Print and shaded views of the part. All mm, measured from the part's lowest x, y and z. A direction names the side the tool comes from. Give positions to 0.01 mm unless a question says otherwise; leave off trailing zeros. Write each loop counter-clockwise with the first axis right and the second up, starting at its lowest first coordinate (ties: lowest second). Pieces come first, ordered by that corner, then holes. Notation, with made-up numbers: (-39.75, -28) - (-13.75, -28) arc R21 ccw to (-13.75, -3) - close; hole circle Ø5 at (1, 78). An arc over 180 degrees is marked (long way). Use one line per item in the form item = value. Start each with the question number.
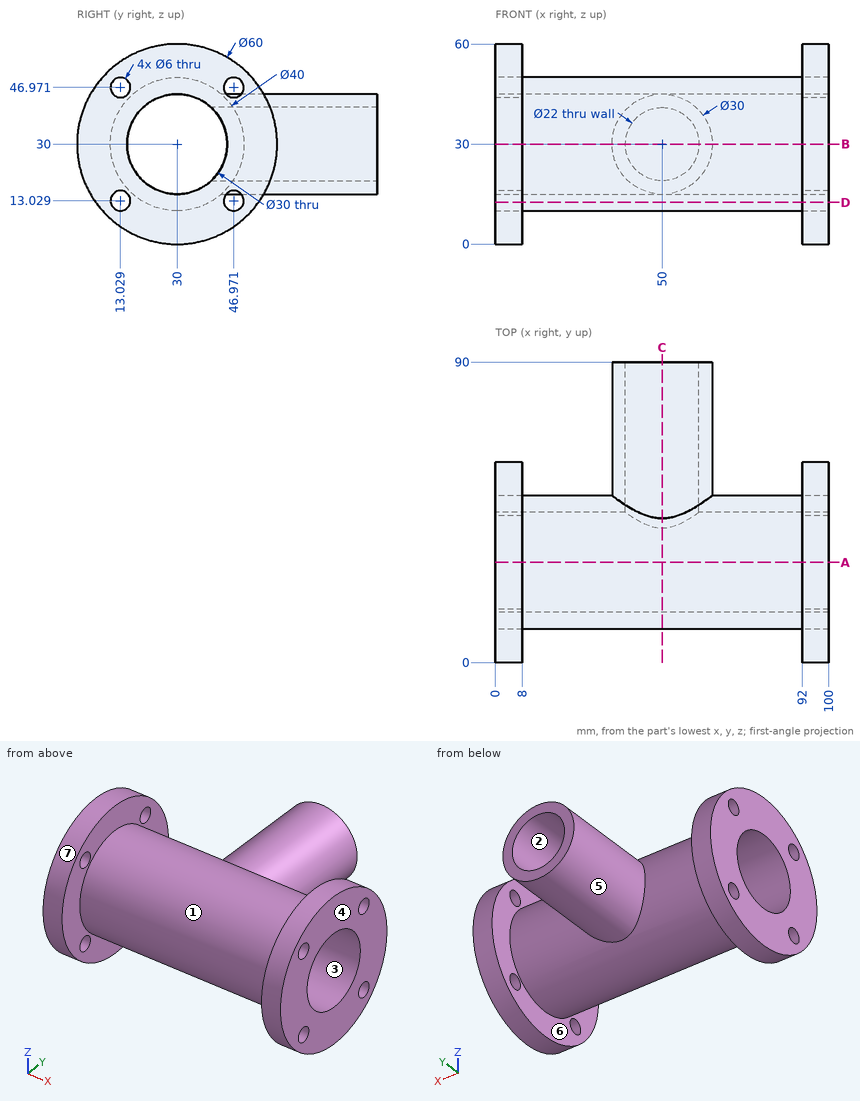
(1) Pin check, flat tips, straight feed: pin 1 Ø4 at (x, z) = (22, 39.5) entering from -Y; pin 2 Ø12 at (x, z) = (24, 39) entering from -Y; pin 3 Ø1.5 at (x, z) = (82.5, 40.5) entering from -Y. Stop position of each tip, or through.
(2) Wall check: line 1 (X direction, y = 48, z = 30.5); line 2 (Y direction, x = 89, z = 30.5); line 3 (X direction, y = 53.5, z = 25). Give the ranges that are in metal, low to high. Write a range as from..to.
(3) Cut at C-C, the plane x = 50. Give the cut face in (y, z).
(4) Cut at A-A, the plane y = 30. Give the cut face in (x, z), then the cut area to 3 significant figures.
(5) Which spindle directions (+Z, -Z, +X, -X, +Y, -Y) get a long thin tool onto all of the face, cutting with end or side? Do the marked faces 1, 2 and 3. Say none if no direction does.
(6) Cut at D-D, the plane z = 12.5. Give the cut face in (x, y), then the cut area to 3 significant figures.
(7) Cut at B-B, the plane z = 30. Give the cut face in (x, y), then the cut area to 3 significant figures.
(8) Two-plate mould, pull along X, no slides. Class the marked faces 4, 5, 6 and 7: +X half, -X half, draft (parallel to the pull), parting line (faces both ways), or undercut.
Solution:
q1.pin_1 = 11.46
q1.pin_2 = 10.23
q1.pin_3 = 12.54
q2.line_1 = 0..39.01, 60.99..100
q2.line_2 = 10.01..15.01, 44.99..49.99
q2.line_3 = 0..8, 35.86..40.2, 59.8..64.14, 92..100
q3.outline = (40.2, 19) arc R15 cw (long way) to (40.2, 41) - (90, 41) - (90, 45) - (43.23, 45) arc R20 ccw (long way) to (43.23, 15) - (90, 15) - (90, 19) - close
q4.outline = (0, 0) - (8, 0) - (8, 10) - (92, 10) - (92, 0) - (100, 0) - (100, 15) - (0, 15) - close; (0, 45) - (100, 45) - (100, 60) - (92, 60) - (92, 50) - (8, 50) - (8, 60) - (0, 60) - close
q4.area = 1,320 mm2
q5.face_1 = none
q5.face_2 = +Y
q5.face_3 = +X, -X
q6.outline = (0, 5.63) - (8, 5.63) - (8, 10.08) - (0, 10.08) - close; (0, 15.98) - (8, 15.98) - (8, 20.32) - (92, 20.32) - (92, 15.98) - (100, 15.98) - (100, 44.02) - (92, 44.02) - (92, 39.68) - (8, 39.68) - (8, 44.02) - (0, 44.02) - close; (0, 49.92) - (8, 49.92) - (8, 54.37) - (0, 54.37) - close; (92, 5.63) - (100, 5.63) - (100, 10.08) - (92, 10.08) - close; (92, 49.92) - (100, 49.92) - (100, 54.37) - (92, 54.37) - close
q6.area = 2,220 mm2
q7.outline = (0, 0) - (8, 0) - (8, 10) - (92, 10) - (92, 0) - (100, 0) - (100, 15) - (0, 15) - close; (0, 45) - (39, 45) - (39, 90) - (35, 90) - (35, 50) - (8, 50) - (8, 60) - (0, 60) - close; (61, 45) - (100, 45) - (100, 60) - (92, 60) - (92, 50) - (65, 50) - (65, 90) - (61, 90) - close
q7.area = 1,530 mm2
q8.face_4 = +X half
q8.face_5 = undercut
q8.face_6 = undercut
q8.face_7 = draft
